Answer from the drawing. Dimensions are ordinates in mm from the lowest x, y and z of the part. A direction names the side the tool comes from. Coordinates: 2 decimals unless noted, no trailing zeros. Loops run counter-clockwise (first coordinate to the right, second up) from the corner with the lowest first, then second, coordinate; pieces in that order, holes last. Notation, with made-up numbers: M 9,-32.5 L 15,-32.5 A28 cw 15,5.5 Z; hole C -29,88 d3. An arc over 180 degrees is marked long. Answer as CSV lines item,"result". Start each with the question number.
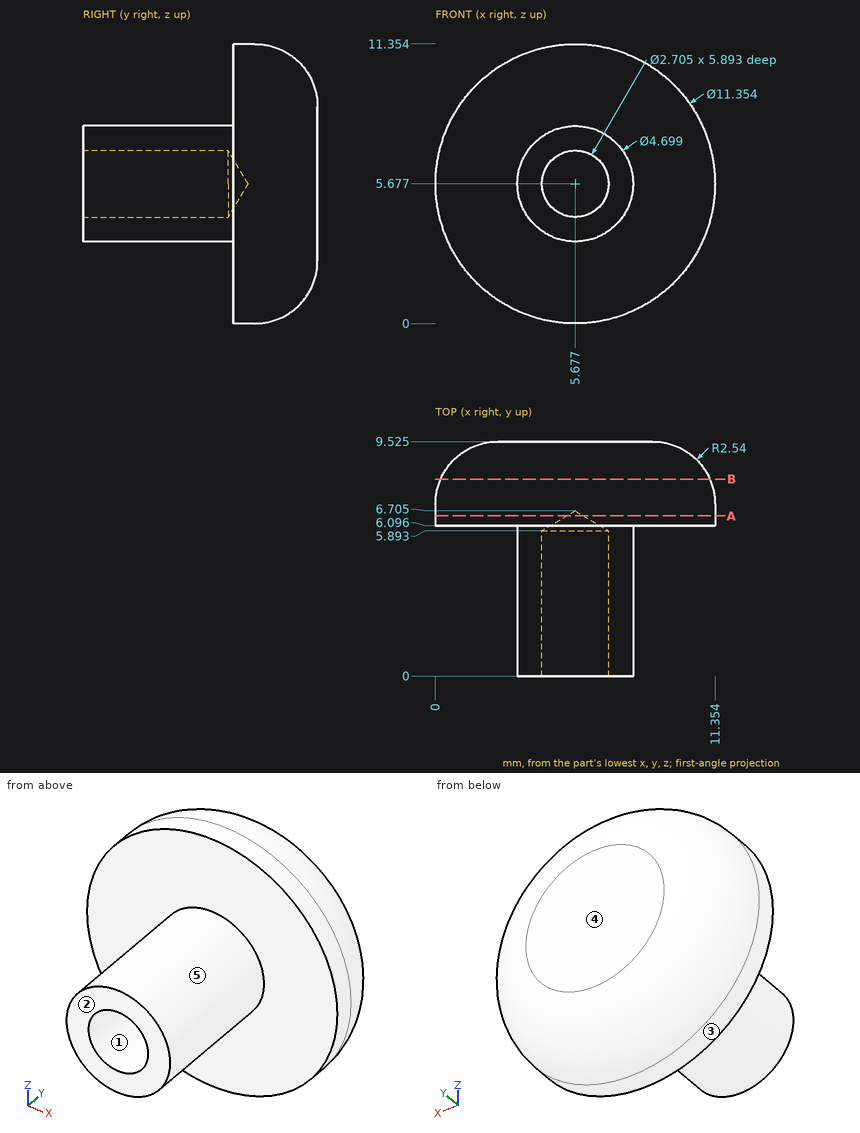
Item 1: Section B-B on y = 8 is taken. Determine the outline of the cut face in (x, z) (1 decimal).
Item 2: Each of these flat-tipped pins is pushed along its axis until it touches: P1, Ø4, axis at x = 7, y = 2, coming from the -Z side; P2, Ø2, axis at x = 8, y = 4, coming from the +Z side; P3, Ø4, axis at y = 3, z = 3, coming from the +X side. Where does it stop, or does it pass through?
Item 3: For the marked faces 4 and 5, determine the directions among +Z, -Z, +X, -X, +Y, -Y from which every point of the face is accessible in a straight line to the end or side of a thin tool.
Item 4: For a pull along X with two mould halves and no side action, classify the marked faces 1, 2 and 3 as pulls with the +X half, pulls with the -X half, needs draft (parallel to the pull), parting line crosses it, or undercut.
Item 5: Consider line 1 (Y direction, x = 4.5, z = 8.5) (1 decimal); line 2 (Y direction, x = 6, z = 6) (1 decimal); line 3 (Z direction, x = 5.5, y = 4.5) (1 decimal). Determine where each line is inside the solid, lowest interval first.
Item 6: Section A-A on y = 6.5 is taken. Determine the outline of the cut face in (x, z), then the cut area to 3 significant figures.
Results are:
1,outline,"C 5.7,5.7 d10.9"
2,P1,"z = 3.33"
2,P2,"z = 7.62"
2,P3,"x = 7.93"
3,face 4,"+Z, -Z, +X, -X, +Y"
3,face 5,"-Y"
4,face 1,"undercut"
4,face 2,"needs draft"
4,face 3,"parting line crosses it"
5,line 1,"6.1 to 9.5"
5,line 2,"6.4 to 9.5"
5,line 3,"3.3 to 4.3, 7 to 8"
6,outline,"C 5.68,5.68 d11.35; hole C 5.68,5.68 d0.68"
6,area,"101 mm²"
